Work out the finished part from the listing and answer in its coordinate system (mm). A direction names the side the tool comes from. Coordinates: 2 decimals unless noted, no trailing zeros. Order: outer loops, then holes, each group sorted by start corner. A loop starts at its lowest first (then second) coordinate and runs counter-clockwise, first axis right, second up. Notation, with made-up numbers: M 44.25,-15 L 102.25,-15 A17 cw 102.25,-11 Z; hole C 60,3 d6. An arc over 180 degrees is marked long. Use a Markdown table: item, result. Add a question column.
from build123d import *

# Parameters (mm, degrees)
PAD_DEPTH       = 20
SKETCH001_R     = 2.25
POCKET_DEPTH    = 7.001
SKETCH002_R     = 4
POCKET001_DEPTH = 5
CHAMFER_SIZE    = 1.5
FILLET_R        = 1
FILLET001_R     = 1


with BuildPart() as part:
    # Sketch (on XY_Plane of Origin) → Pad (new body)
    with BuildSketch(Plane.XY):
        Polygon((-19.5, 0), (-19.5, 5), (-9.5, 5), (-5, 11), (5, 11), (9.5, 5), (19.5, 5), (19.5, 0), (2.46556, 0), (2.46556, 7), (-2.53444, 7), (-2.46556, 0), align=None)
    extrude(amount=PAD_DEPTH)

    # Sketch001 → Pocket (cut, through all)
    with BuildSketch(Plane(origin=(0, 7, 0), x_dir=(-1, 0, 0), z_dir=(0, 1, 0))):
        with Locations((-13.21875, 10)):
            Circle(SKETCH001_R)
        with Locations((13.21875, 10)):
            Circle(SKETCH001_R)
    extrude(amount=-POCKET_DEPTH, mode=Mode.SUBTRACT)

    # Sketch002 (on Face6 of Pocket) → Pocket001 (cut)
    with BuildSketch(Plane(origin=(0, 5, 0), x_dir=(-1, 0, 0), z_dir=(0, 1, 0))):
        with Locations((-13.21875, 10)):
            Circle(SKETCH002_R)
        with Locations((13.21875, 10)):
            Circle(SKETCH002_R)
    extrude(amount=POCKET001_DEPTH, mode=Mode.SUBTRACT)

    # Chamfer
    chamfer_edges = [part.edges().sort_by_distance(p)[0] for p in [
        (-10.96875, 5, 10),
        (15.46875, 5, 10),
    ]]
    chamfer(chamfer_edges, length=CHAMFER_SIZE)

    # Fillet
    fillet_edges = [part.edges().sort_by_distance(p)[0] for p in [
        (-19.5, 5, 10),
        (-5, 11, 10),
        (5, 11, 10),
        (19.5, 5, 10),
    ]]
    fillet(fillet_edges, radius=FILLET_R)

    # Fillet001
    fillet001_edges = [part.edges().sort_by_distance(p)[0] for p in [
        (-14, 5, 20),
        (-14, 5, 0),
        (-7.4, 7.8, 0),
        (0, 11, 0),
        (7.4, 7.8, 0),
        (14, 5, 0),
        (14, 5, 20),
        (7.4, 7.8, 20),
        (0, 11, 20),
        (-7.4, 7.8, 20),
    ]]
    fillet(fillet001_edges, radius=FILLET001_R)


solid = part.part
(1) A cutting plane is placed at A-A on z = 10. Count the separate pieces of the cut face and the enclosed holes in it, plus the area to 3 significant figures.
(2) A cutting plane is placed at B-B on y = 0.5. Write down the section's boundary in (x, z).
(3) Which of the six approach directions +Z, -Z, +X, -X, +Y, -Y give full straight-line access (tool end or side, diameter ignored) to faces 1 (the cylindrical face through (-13.683, 4.699, 0.285)), 2 (the cylindrical face through (-13.683, 4.699, 19.715)), 3 (the flat face through (2.466, 3, 10)), 4 (the cylindrical face through (19.215, 1.972, 0.301)), 5 (the cylindrical face through (-19.199, 2.028, 0.285))?
(4) Given P1, Ø12, axis at x = 13, z = 13, coming from the -Y side; P2, Ø7.5, axis at x = -15, z = 6, coming from the +Y side; P3, Ø1.5, axis at x = -1, z = 12, coming from the -Y side; P4, Ø1.5, axis at y = 6.5, z = 9.5, coming from the +X side, each flat-ended and moving along its own axis, determine where each tip first touches the part or whether it passes through.
(5) A cutting plane is placed at C-C on z = 17. Write down the section's boundary in (x, y).
(6) Straight lines are drawn through the part: line 1 (Y direction, x = 17.5, z = 13.75); line 2 (Y direction, x = 6.5, z = 2); line 3 (X direction, y = 4.25, z = 14.75). For each, find the intervals that lie inside material, in ascending order.
(7) A cutting plane is placed at D-D on x = -1. Write down the section's boundary in (y, z).
From the geometry:
| question | item | result |
|---|---|---|
| 1 | separate pieces | 3 |
| 1 | enclosed holes | 0 |
| 1 | area | 197 mm2 |
| 2 | outline | M -19.5,1 A1 ccw -18.5,0 L -2.47,0 L -2.47,20 L -18.5,20 A1 ccw -19.5,19 Z; M 2.47,0 L 18.5,0 A1 ccw 19.5,1 L 19.5,19 A1 ccw 18.5,20 L 2.47,20 Z; hole C -13.22,10 d4.5; hole C 13.22,10 d4.5 |
| 3 | face 1 | -Z, -X, +Y |
| 3 | face 2 | +Z, -X, +Y |
| 3 | face 3 | +Z, -Z, -Y |
| 3 | face 4 | -Z, +X, +Y, -Y |
| 3 | face 5 | -Z, -X, +Y, -Y |
| 4 | P1 | stops at y = 0 |
| 4 | P2 | stops at y = 5 |
| 4 | P3 | stops at y = 7 |
| 4 | P4 | stops at x = 8.94 |
| 5 | outline | M -19.5,0 L -2.47,0 L -2.53,7 L 2.47,7 L 2.47,0 L 19.5,0 L 19.5,4 A1 ccw 18.5,5 L 9.5,5 L 5.3,10.6 A1 ccw 4.5,11 L -4.5,11 A1 ccw -5.3,10.6 L -9.5,5 L -18.5,5 A1 ccw -19.5,4 Z |
| 6 | line 1 | y = 0 to 5 |
| 6 | line 2 | y = 0 to 9 |
| 6 | line 3 | x = -19.47 to -2.51, 2.47 to 19.47 |
| 7 | outline | M 7,0 L 10,0 A1 ccw 11,1 L 11,19 A1 ccw 10,20 L 7,20 Z |
